Design review of the part shown in the three views and the two pictorial views. Dimensions are in mm from the part's minimum x, y and z. Round coordinates to 2 decimals unless told otherwise and drop trailing zeros. Write each loop counter-clockwise with the first axis right and the second up, starting at its lowest first coordinate (ties: lowest second). Pieces come first, ordered by that corner, then holes. Notation, with made-up numbers: (-35, -16) - (12, -16) arc R27 ccw to (12, 17) - close; hole circle Ø11 at (-2, 41). An arc over 180 degrees is marked (long way). Use one line per item in the form item = value.
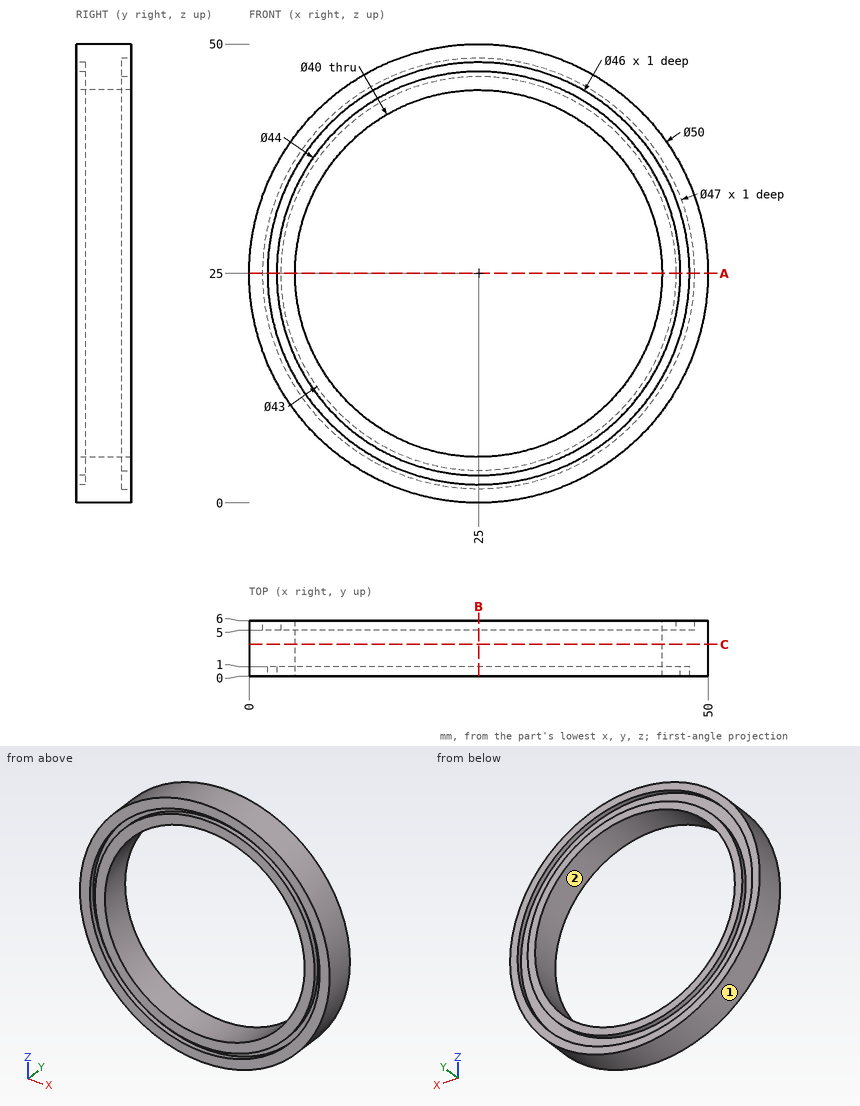
(1) The part is to be moulded in two halves that separate along X. For the marked faces 1 and 2, say which applies: +X half, -X half, draft (parallel to the pull), parting line (faces both ways), or undercut.
Geometry results:
face_1 = parting line
face_2 = undercut
(2) Add section A-A on z = 25. Write out the cut boundary in (x, y), then the cut area to 3 significant figures.
Geometry results:
outline = (0, 0) - (2, 0) - (2, 1) - (3, 1) - (3, 0) - (5, 0) - (5, 6) - (3.5, 6) - (3.5, 5) - (1.5, 5) - (1.5, 6) - (0, 6) - close; (45, 0) - (47, 0) - (47, 1) - (48, 1) - (48, 0) - (50, 0) - (50, 6) - (48.5, 6) - (48.5, 5) - (46.5, 5) - (46.5, 6) - (45, 6) - close
area = 54.0 mm2
(3) Add section B-B on x = 25. Write out the cut boundary in (y, z), then the cut area to 3 significant figures.
Geometry results:
outline = (0, 0) - (6, 0) - (6, 1.5) - (5, 1.5) - (5, 3.5) - (6, 3.5) - (6, 5) - (0, 5) - (0, 3) - (1, 3) - (1, 2) - (0, 2) - close; (0, 45) - (6, 45) - (6, 46.5) - (5, 46.5) - (5, 48.5) - (6, 48.5) - (6, 50) - (0, 50) - (0, 48) - (1, 48) - (1, 47) - (0, 47) - close
area = 54.0 mm2
(4) Add section C-C on y = 3.45. Write out the cut boundary in (x, z), then the cut area to 3 significant figures.
Geometry results:
outline = circle Ø50 at (25, 25); hole circle Ø40 at (25, 25)
area = 707 mm2
(5) To check wall thickness, follow L1, parallel to X at y = 5.5, z = 25; L2, parallel to Z at x = 25, y = 0.5; L3, parallel to Z at x = 25, y = 2. State the ranges of each line that lie inside material, in increasing order.
Geometry results:
L1 = 0 to 1.5, 3.5 to 5, 45 to 46.5, 48.5 to 50
L2 = 0 to 2, 3 to 5, 45 to 47, 48 to 50
L3 = 0 to 5, 45 to 50
(6) Insertion check: P1, Ø1.5, axis at x = 18.5, y = 1.5, coming from the -Z side; P2, Ø14, axis at x = 15.5, z = 25, coming from the +Y side; P3, Ø2, axis at y = 5, z = 15, coming from the -X side; P4, Ø3, axis at y = 3, z = 20.5, coming from the +X side. Each pin has a flat end and moves straight along its axis. Give the tip position at first contact, or say it passes through.
Geometry results:
P1 = 0.67
P2 = through
P3 = 1.68
P4 = 49.82
